Could you check a few things on this drawing? It's one solid part, dimensions in mm from its lowest x, y, z. A direction names the side the tool comes from. Give positions to 0.01 mm unless a question says otherwise; leave off trailing zeros. Order: outer loops, then holes, each group sorted by start corner. A loop starts at its lowest first (then second) coordinate and runs counter-clockwise, first axis right, second up. Notation, with made-up numbers: (50.25, 46.25) - (75.25, 46.25) arc R11 cw to (75.25, 57.25) - close; hole circle Ø11 at (-23.75, 67). An arc over 180 degrees is marked (long way). One line per question, with ' | ' between items. Start each with the question number.
1. Imagine slicing it at A-A (z = 11). Please give me the cut outline in (x, y).
2. Imagine slicing it at C-C (x = 14.5). Please give me the cut outline in (y, z).
3. Imagine slicing it at D-D (y = 39.5). Please give me the cut outline in (x, z).
4. I need wall thicknesses on probe 1 along X at (y, z) = (26, 30.5); probe 2 along Z at (x, y) = (44.5, 3). Which ranges of each line are inside material? Lowest first, please. Write a range as from..to.
5. For P1, Ø5, axis at y = 23.5, z = 36, coming from the -X side; P2, Ø1.2, axis at x = 1, z = 25.5, coming from the +Y side; P3, Ø10, axis at x = 57.5, y = 16, coming from the +Z side, each with a flat end and sliding along its axis, tell me the tip position at first contact or that it passes through.
6. Which directions (+Z, -Z, +X, -X, +Y, -Y) give clear straight access to the entire face, cutting with the end or side of a thin tool? Please do the marked faces 1 and 2.
7. If we mould it in two halves opening along X, with no side actions, what happens to the marked faces 3, 4, 5 and 6? For each: released by +X, released by -X, zero draft, split by the parting line, or undercut.
8. Imagine slicing it at B-B (y = 19). Please give me the cut outline in (x, z), and give its area (3 significant figures).
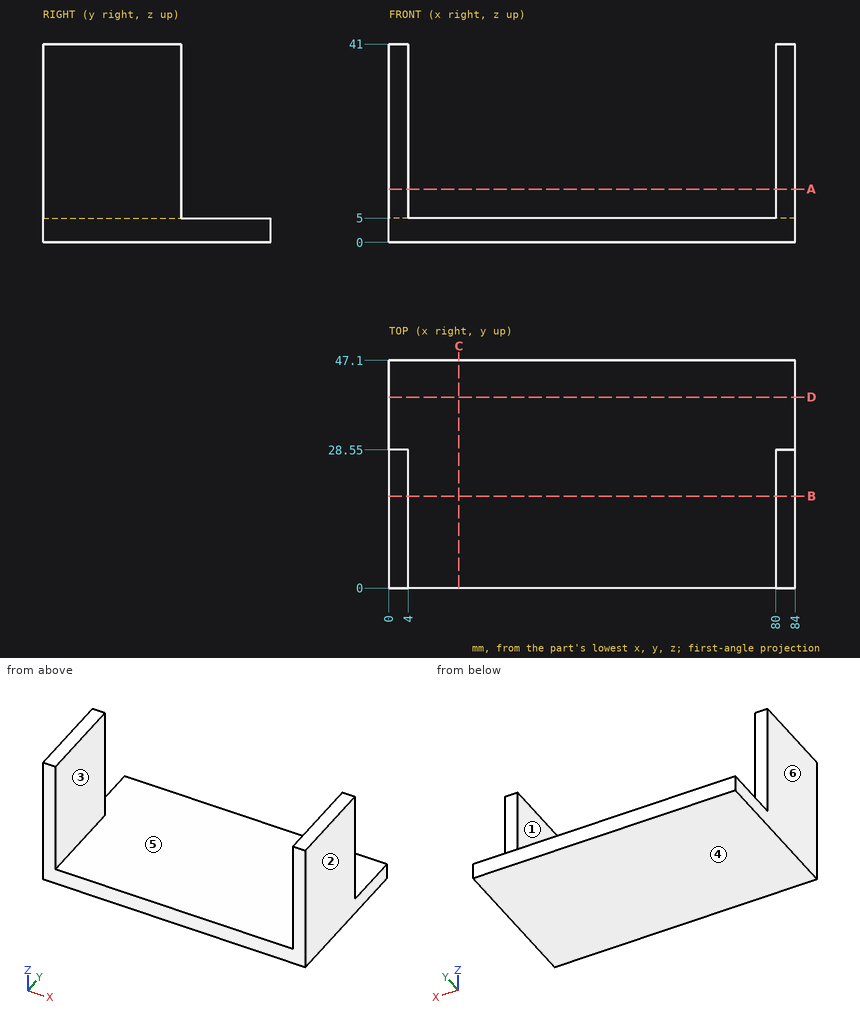
Results found:
1) outline: (0, 0) - (4, 0) - (4, 28.55) - (0, 28.55) - close; (80, 0) - (84, 0) - (84, 28.55) - (80, 28.55) - close
2) outline: (0, 0) - (47.1, 0) - (47.1, 5) - (0, 5) - close
3) outline: (0, 0) - (84, 0) - (84, 5) - (0, 5) - close
4) probe 1: x = 0..4, 80..84 | probe 2: z = 0..5
5) P1: stops at x = 0 | P2: stops at y = 28.55 | P3: stops at z = 5
6) face 1: +Z, +Y, -Y | face 2: +Z, -Z, +X, +Y, -Y
7) face 3: undercut | face 4: zero draft | face 5: undercut | face 6: released by -X
8) outline: (0, 0) - (84, 0) - (84, 41) - (80, 41) - (80, 5) - (4, 5) - (4, 41) - (0, 41) - close | area: 708 mm2
